```python
from build123d import *

# Parameters (mm, degrees)
BOSS_EXTRUDE1_DEPTH          = 8
CUT_EXTRUDE2_DEPTH           = 1.2
CUT_EXTRUDE3_DEPTH           = 10.965900881
FILLET1_R                    = 1
M2_2X0_45_TAPPED_HOLE1_D     = 1.75
M2_2X0_45_TAPPED_HOLE1_DEPTH = 3.474246958
M2_2X0_45_TAPPED_HOLE1_TIP   = 0.525753042
CUT_EXTRUDE4_DEPTH           = 10.965900881


with BuildPart() as part:
    # Sketch1 → Boss-Extrude1 (new body, symmetric)
    with BuildSketch(Plane(origin=(0, 0, 0), x_dir=(0, 0, -1), z_dir=(1, 0, 0))):
        Polygon((13, 0), (-13, 0), (-13.522642316, 4.972609477), (11.954212859, 9.95), align=None)
    extrude(amount=BOSS_EXTRUDE1_DEPTH, both=True)

    # Sketch2 → Cut-Extrude2 (cut)
    with BuildSketch(Plane(origin=(0, 7.334562502, 1.432946949), x_dir=(1, 0, 0), z_dir=(0, 0.981444969, 0.19174403))):
        with BuildLine():
            Line((-5.7, -12.995337767), (-5.7, 8.740255167))
            ThreePointArc((-5.7, 8.740255167), (-2.2, 12.240255167), (1.3, 8.740255167))
            Line((1.3, 8.740255167), (1.3, -12.995337767))
            Line((1.3, -12.995337767), (-5.7, -12.995337767))
        make_face()
    extrude(amount=-CUT_EXTRUDE2_DEPTH, mode=Mode.SUBTRACT)

    # Sketch5 → Cut-Extrude3 (cut, through all)
    with BuildSketch(Plane(origin=(0, 7.334562502, 1.432946949), x_dir=(1, 0, 0), z_dir=(0, 0.981444969, 0.19174403))):
        with BuildLine():
            Line((-8, 6.140255167), (-8, -4.818261086))
            ThreePointArc((-8, -4.818261086), (-6.5, 0.660997041), (-8, 6.140255167))
        make_face()
        with BuildLine():
            Line((8, 6.140255167), (8, -4.818261086))
            ThreePointArc((8, -4.818261086), (6.5, 0.660997041), (8, 6.140255167))
        make_face()
    extrude(amount=-CUT_EXTRUDE3_DEPTH, mode=Mode.SUBTRACT)

    # Fillet1
    fillet1_edges = [part.edges().sort_by_distance(p)[0] for p in [
        (8, 2.486304738, 13.261321158),
        (8, 4.975, -12.47710643),
        (-8, 2.486304738, 13.261321158),
        (-8, 4.975, -12.47710643),
    ]]
    fillet(fillet1_edges, radius=FILLET1_R)

    # Sketch6 → Cut-Revolve1 (revolve, cut)
    with BuildSketch(Plane(origin=(2, 0, 0), x_dir=(0, 0, -1), z_dir=(1, 0, 0))):
        Polygon((13.04508728, 9.137795416), (-14.42511425, 3.992284126), (-14.282095982, 2.631556203), (-14.256713544, 2.390058443), (13.472498816, 5.071246296), align=None)
    revolve(axis=Axis((2, 2.390058443, 14.256713544), (0, 0.096242959, -0.995357872)), mode=Mode.SUBTRACT)

    # M2.2x0.45 Tapped Hole1
    with Locations(Plane(origin=(0, 6.156828539, 1.202854113), x_dir=(1, 0, 0), z_dir=(0, 0.981444969, 0.19174403))):
        with Locations((-2.9, -0.424399477)):
            Hole(M2_2X0_45_TAPPED_HOLE1_D / 2, depth=M2_2X0_45_TAPPED_HOLE1_DEPTH)
            with Locations((0, 0, -(M2_2X0_45_TAPPED_HOLE1_DEPTH + M2_2X0_45_TAPPED_HOLE1_TIP / 2))):  # 118° drill point
                Cone(0, M2_2X0_45_TAPPED_HOLE1_D / 2, M2_2X0_45_TAPPED_HOLE1_TIP, mode=Mode.SUBTRACT)

    # Sketch9 → Cut-Extrude4 (cut, through all)
    with BuildSketch(Plane(origin=(0, 7.334562502, 1.432946949), x_dir=(1, 0, 0), z_dir=(0, 0.981444969, 0.19174403))):
        with BuildLine():
            ThreePointArc((-7.289795354, 5.159702376), (-7.451242382, 5.201326159), (-7.563470071, 5.324625097))
            ThreePointArc((-7.563470071, 5.324625097), (-7.252547552, 4.613795693), (-6.993667337, 3.882405038))
            ThreePointArc((-6.993667337, 3.882405038), (-7.004481287, 4.117448052), (-6.897853081, 4.327192148))
            ThreePointArc((-6.897853081, 4.327192148), (-6.818575776, 4.873033057), (-7.289795354, 5.159702376))
        make_face()
        with BuildLine():
            ThreePointArc((-6.660871352, 3.572142615), (-6.868230387, 3.683337889), (-6.993667337, 3.882405038))
            ThreePointArc((-6.993667337, 3.882405038), (-6.776841479, 3.085777587), (-6.621748536, 2.274867649))
            ThreePointArc((-6.621748536, 2.274867649), (-6.596489986, 2.508799625), (-6.459039737, 2.69976976))
            ThreePointArc((-6.459039737, 2.69976976), (-6.289708944, 3.198480265), (-6.660871352, 3.572142615))
        make_face()
        with BuildLine():
            ThreePointArc((-6.340315921, 1.917360153), (-6.528230594, 2.05895899), (-6.621748536, 2.274867649))
            ThreePointArc((-6.621748536, 2.274867649), (-6.529302038, 1.454451661), (-6.500046516, 0.629362053))
            ThreePointArc((-6.500046516, 0.629362053), (-6.439309701, 0.856679466), (-6.274271086, 1.024382842))
            ThreePointArc((-6.274271086, 1.024382842), (-6.030663985, 1.491331089), (-6.340315921, 1.917360153))
        make_face()
        with BuildLine():
            ThreePointArc((-6.2765983, 0.23302027), (-6.440647698, 0.401691388), (-6.500046516, 0.629362053))
            ThreePointArc((-6.500046516, 0.629362053), (-6.534154287, -0.195541178), (-6.631424447, -1.015399212))
            ThreePointArc((-6.631424447, -1.015399212), (-6.536638256, -0.80004432), (-6.347894026, -0.659553155))
            ThreePointArc((-6.347894026, -0.659553155), (-6.035741762, -0.235352673), (-6.2765983, 0.23302027))
        make_face()
        with BuildLine():
            ThreePointArc((-6.47121752, -1.441250956), (-6.607542206, -1.249475706), (-6.631424447, -1.015399212))
            ThreePointArc((-6.631424447, -1.015399212), (-6.791284069, -1.825382978), (-7.012791541, -2.620721422))
            ThreePointArc((-7.012791541, -2.620721422), (-6.886185953, -2.422395441), (-6.678176493, -2.312421653))
            ThreePointArc((-6.678176493, -2.312421653), (-6.304822815, -1.940948752), (-6.47121752, -1.441250956))
        make_face()
        with BuildLine():
            ThreePointArc((-6.919594936, -3.066064322), (-7.024987686, -2.855696746), (-7.012791541, -2.620721422))
            ThreePointArc((-7.012791541, -2.620721422), (-7.264215038, -3.321206437), (-7.563470071, -4.002631015))
            ThreePointArc((-7.563470071, -4.002631015), (-7.47948201, -3.914560625), (-7.359806711, -3.892465134))
            ThreePointArc((-7.359806711, -3.892465134), (-6.85334699, -3.631801278), (-6.919594936, -3.066064322))
        make_face()
        with BuildLine():
            ThreePointArc((7.563470071, -4.002631015), (7.264215036, -3.321206432), (7.012791537, -2.620721412))
            ThreePointArc((7.012791537, -2.620721412), (7.024987687, -2.855696741), (6.919594936, -3.066064322))
            ThreePointArc((6.919594936, -3.066064322), (6.85334699, -3.631801278), (7.359806711, -3.892465134))
            ThreePointArc((7.359806711, -3.892465134), (7.47948201, -3.914560625), (7.563470071, -4.002631015))
        make_face()
        with BuildLine():
            ThreePointArc((7.012791537, -2.620721412), (6.791284072, -1.825382992), (6.631424452, -1.01539925))
            ThreePointArc((6.631424452, -1.01539925), (6.607542199, -1.249475724), (6.47121752, -1.441250956))
            ThreePointArc((6.47121752, -1.441250956), (6.304822815, -1.940948752), (6.678176493, -2.312421653))
            ThreePointArc((6.678176493, -2.312421653), (6.886185949, -2.422395438), (7.012791537, -2.620721412))
        make_face()
        with BuildLine():
            ThreePointArc((6.631424452, -1.01539925), (6.534154286, -0.195541171), (6.500046515, 0.629362105))
            ThreePointArc((6.500046515, 0.629362105), (6.440647711, 0.401691411), (6.2765983, 0.23302027))
            ThreePointArc((6.2765983, 0.23302027), (6.035741762, -0.235352673), (6.347894026, -0.659553155))
            ThreePointArc((6.347894026, -0.659553155), (6.536638268, -0.800044334), (6.631424452, -1.01539925))
        make_face()
        with BuildLine():
            ThreePointArc((6.500046515, 0.629362105), (6.52930204, 1.454451696), (6.621748538, 2.274867666))
            ThreePointArc((6.621748538, 2.274867666), (6.528230599, 2.058958996), (6.340315921, 1.917360153))
            ThreePointArc((6.340315921, 1.917360153), (6.030663985, 1.491331089), (6.274271086, 1.024382842))
            ThreePointArc((6.274271086, 1.024382842), (6.439309688, 0.856679489), (6.500046515, 0.629362105))
        make_face()
        with BuildLine():
            ThreePointArc((6.621748538, 2.274867666), (6.776841483, 3.085777604), (6.993667342, 3.882405056))
            ThreePointArc((6.993667342, 3.882405056), (6.868230394, 3.683337895), (6.660871352, 3.572142615))
            ThreePointArc((6.660871352, 3.572142615), (6.289708944, 3.198480265), (6.459039737, 2.69976976))
            ThreePointArc((6.459039737, 2.69976976), (6.596489983, 2.508799632), (6.621748538, 2.274867666))
        make_face()
        with BuildLine():
            ThreePointArc((7.563470071, 5.324625097), (7.451242382, 5.201326159), (7.289795354, 5.159702376))
            ThreePointArc((7.289795354, 5.159702376), (6.818575776, 4.873033057), (6.897853081, 4.327192148))
            ThreePointArc((6.897853081, 4.327192148), (7.004481285, 4.117448061), (6.993667342, 3.882405056))
            ThreePointArc((6.993667342, 3.882405056), (7.252547555, 4.613795701), (7.563470071, 5.324625097))
        make_face()
    extrude(amount=-CUT_EXTRUDE4_DEPTH, mode=Mode.SUBTRACT)


solid = part.part
```
Build history of the part. All positions in model axes, mm. A direction names the side the tool comes from. Round coordinates to 2 decimals unless told otherwise and drop trailing zeros.
Item 1: Pin check, flat tips, straight feed: P1, Ø2, axis at x = -4.5, y = 3.5, coming from the +Z side; P2, Ø3, axis at x = -1, y = 5, coming from the -Z side; P3, Ø4, axis at y = 5.5, z = -1, coming from the -X side. Stop position of each tip, or through.
Item 2: Which spindle directions (+Z, -Z, +X, -X, +Y, -Y) get a long thin tool onto all of the face, cutting with end or side? Do faces 5 (the face through (-2.277, 9.101, -10.693)), 6 (the face through (-3.01, 5.04, -12.47)), 7 (the face through (2.125, 0.893, 0.29)). Say none if no direction does.
Item 3: Two-plate mould, pull along Y, no slides. Class faces 1 (the face through (-2.026, 4.354, 1.244)), 2 (the face through (-5.7, 6, 3)), 3 (the face through (7.71, 2.55, 12.97)), 4 (the face through (-7.7, 4.9, -12.2)): released by +Y, released by -Y, zero draft, split by the parting line, or undercut.
Item 4: Drill centre lines: line 1 along X through (y, z) = (5, 10.75); line 2 along X through (y, z) = (7.5, 0); line 3 along Y through (x, z) = (-6.25, 8.25). Where is each one in solid material? Low to high.
Worked answers:
1. P1: stops at z = 13.4
1. P2: stops at z = -12.61
1. P3: stops at x = -7.01
2. face 5: +Z
2. face 6: -Z, +X, -X, +Y
2. face 7: none
3. face 1: undercut
3. face 2: zero draft
3. face 3: released by -Y
3. face 4: released by +Y
4. line 1: x = -8 to -5.7, 1.3 to 8
4. line 2: x = -6.03 to -5.7, 1.3 to 6.03
4. line 3: y = 0 to 6
